Autodesk Inventor part; units mm, degrees
ref_plane "YZ Plane" through (0, 0, 0) normal (1, 0, 0) x (0, 1, 0)
ref_plane "XZ Plane" through (0, 0, 0) normal (0, 1, 0) x (-1, 0, 0)
ref_plane "XY Plane" through (0, 0, 0) normal (0, 0, 1) x (1, 0, 0)
sketch "草图1" plane through (0, 0, 0) normal (0, 1, 0) x (-1, 0, 0)
  line L0 (125, 245) -> (-125, 245)
  line L1 (-125, 245) -> (-125, -245)
  line L2 (-125, -245) -> (125, -245)
  line L3 (125, -245) -> (125, 245)
  line L4 (0, 3) -> (0, -5)
  line L5 (3.5058, 0) -> (-3.4421, 0)
  line L6 (25, 144) -> (-32, 144)
  line L7 (-32, 144) -> (-32, 87)
  line L8 (-32, 87) -> (25, 87)
  line L9 (25, 87) -> (25, 144)
  line L10 (25, 67) -> (-32, 67)
  line L11 (-32, 67) -> (-32, 10)
  line L12 (-32, 10) -> (25, 10)
  line L13 (25, 10) -> (25, 67)
  line L14 (25, -10) -> (-32, -10)
  line L15 (-32, -10) -> (-32, -67)
  line L16 (-32, -67) -> (25, -67)
  line L17 (25, -67) -> (25, -10)
  line L18 (25, -87) -> (-32, -87)
  line L19 (-32, -87) -> (-32, -144)
  line L20 (-32, -144) -> (25, -144)
  line L21 (25, -144) -> (25, -87)
  line L22 (-66, 100) -> (-95, 100)
  line L23 (-95, 100) -> (-95, 54)
  line L24 (-95, 54) -> (-66, 54)
  line L25 (-66, 54) -> (-66, 100)
  line L26 (-66, -54) -> (-95, -54)
  line L27 (-95, -54) -> (-95, -100)
  line L28 (-95, -100) -> (-66, -100)
  line L29 (-66, -100) -> (-66, -54)
  line L30 (100, 15) -> (70, 15)
  line L31 (70, 15) -> (70, -15)
  line L32 (70, -15) -> (100, -15)
  line L33 (100, -15) -> (100, 15)
  circle A0 centre (65, 182) radius 10
  circle A1 centre (65, -182) radius 10
  circle A2 centre (65, 182) radius 15
  circle A3 centre (80, 182) radius 1.5
  circle A4 centre (57.5, 194.9904) radius 1.5
  circle A5 centre (57.5, 169.0096) radius 1.5
  line L34 (125, 245) -> (0, 245)
  line L35 (0, 245) -> (0, 0)
  line L36 (0, 0) -> (125, 0)
  line L37 (125, 0) -> (125, 245)
  line L38 (-125, 245) -> (0, 245)
  line L39 (0, 245) -> (0, 0)
  line L40 (0, 0) -> (-125, 0)
  line L41 (-125, 0) -> (-125, 245)
  line L42 (-125, -245) -> (0, -245)
  line L43 (0, -245) -> (0, 0)
  line L44 (0, 0) -> (-125, 0)
  line L45 (-125, 0) -> (-125, -245)
  line L46 (125, -245) -> (0, -245)
  line L47 (0, -245) -> (0, 0)
  line L48 (0, 0) -> (125, 0)
  line L49 (125, 0) -> (125, -245)
  circle A6 centre (65, -182) radius 15
  circle A7 centre (80, -182) radius 1.5
  circle A8 centre (57.5, -169.0096) radius 1.5
  circle A9 centre (57.5, -194.9904) radius 1.5
  point P0 (0, -144)
  point P1 (100, 0)
  point P2 (70, 0)
  point P3 (0, -10)
  point P4 (0, -67)
  point P5 (0, -87)
  dimension "d33" = 30
  dimension "d36" = 30
  dimension "d2" = 490
  dimension "d3" = 250
  dimension "d4" = 57
  dimension "d5" = 57
  dimension "d6" = 57
  dimension "d7" = 57
  dimension "d8" = 57
  dimension "d9" = 57
  dimension "d10" = 57
  dimension "d11" = 57
  dimension "d12" = 101
  dimension "d13" = 20
  dimension "d14" = 20
  dimension "d15" = 20
  dimension "d16" = 93
  dimension "d17" = 29
  dimension "d18" = 46
  dimension "d19" = 46
  dimension "d20" = 145
  dimension "d21" = 108
  dimension "d22" = 30
  dimension "d23" = 30
  dimension "d24" = 30
  dimension "d25" = 25
  dimension "d26" = 230
  dimension "d27" = 20
  dimension "d28" = 63
  dimension "d29" = 60
  dimension "d30" = 20
  dimension "d31" = 63
  dimension "d32" = 60
  dimension "d34" = 3
  dimension "d35" = 360
  dimension "d37" = 3
  dimension "d40" = 360
extrude "拉伸1" add sketch "草图1" along normal blind 10 contours L3 L2 L43 L20 L21 L18 L16 L17 L14 L4 L5 L36 L31 L32 L33 | A7 A6 A9 A8
sketch "草图2" plane through (0, 0, 0) normal (0, -1, 0) x (1, 0, 0)
  line L0 (-70, 0) -> (0, 0)
  line L1 (-115, -30) -> (-55, -30)
  line L2 (-55, -30) -> (-55, 0)
  line L3 (-55, 0) -> (-115, 0)
  line L4 (-115, 0) -> (-115, -30)
  line L5 (-100, -15) -> (-70, -15)
  line L6 (-100, 0) -> (-100, -15)
  line L7 (-70, -15) -> (-70, 0)
  line L8 (-40, -159) -> (0, -159)
  line L9 (0, -159) -> (0, 0)
  line L10 (0, 0) -> (-40, 0)
  line L11 (-40, 0) -> (-40, -159)
  line L12 (-25, -10) -> (-25, -67)
  line L13 (-25, -144) -> (0, -144)
  circle A0 centre (-65, -182) radius 10
  circle A1 centre (-65, -182) radius 20
  dimension "d44" = 15
  dimension "d45" = 15
  dimension "d46" = 15
  dimension "d47" = 15
  dimension "d48" = 15
  dimension "d49" = 40
extrude "拉伸2" cut sketch "草图2" against normal blind 5 contours L0 L9 L8 L11 | L0 L2 L1 L4 L3 L6 L5 L7 | A1
sketch "草图5" plane through (0, 10, 0) normal (0, 1, 0) x (1, 0, 0)
  line L0 (0, 159) -> (-40, 159)
  line L1 (0, 159) -> (8, 159)
  line L2 (8, 159) -> (8, 245)
  line L3 (8, 245) -> (0, 245)
  line L4 (0, 245) -> (0, 159)
  circle A0 centre (4, 179) radius 2
  circle A1 centre (4, 225) radius 2
  point P0 (0, 0)
  dimension "d64" = 8
  dimension "d65" = 4
  dimension "d67" = 4
  dimension "d68" = 4
  dimension "d70" = 4
  dimension "d73" = 20
  dimension "d76" = 20
extrude "拉伸4" add sketch "草图5" against normal blind 5
properties part number "top_2"
Here's how the part is built. I have some questions about the finished solid (model axes, mm). A direction names the side the tool comes from. Coordinates: 2 decimals unless noted, no trailing zeros. Write each loop counter-clockwise with the first axis right and the second up, starting at its lowest first coordinate (ties: lowest second). Pieces come first, ordered by that corner, then holes.
Item 1: I want a section at A-A on x = -6. Write out the boundary of the cut face in (y, z), and give its area (4 significant figures).
Item 2: Will these pins go through, and if not, where does the flat tip stop? pin 1 (2.5 mm diameter, centred on x = -57.5, z = -169.01, fed in from +Y); pin 2 (5.5 mm diameter, centred on y = 8, z = -4, fed in from +X); pin 3 (1.5 mm diameter, centred on y = 2, z = -22, fed in from +X); pin 4 (5 mm diameter, centred on x = 4, z = -179, fed in from -Y).
Item 3: If I drill on line 1 (X direction, y = 7.95, z = -182); line 2 (Z direction, x = 4, y = 6.65); line 3 (Z direction, x = -80, y = 8.6), over which ranges is the centre line in solid material (lowest first)?
Item 4: I want a section at C-C on y = 8. Write out the boundary of the cut face in (x, z), and give its area (3 significant figures).
Item 5: On a 3-axis mill with a long thin cutter (end or side, diameter ignored), from which of +Z, -Z, +X, -X, +Y, -Y can I reach the whole of each face in a straight line? I mean faces 5 (the flat face through (0, 7, -152)), 6 (the flat face through (-70, 7, -7)), 7 (the flat face through (-115, 2, -15)), 8 (the cylindrical face through (-67.6, 2.46, -162.17)). Say none if no direction works.
Item 6: If we mould it in two halves opening along Z, with no side actions, what happens to faces 1 (the flat face through (-25, 5, -78)), 2 (the flat face through (-20, 2, -159)), 3 (the flat face through (-25, 7, -116)), 4 (the flat face through (-13, 7, -87))? For each: +Z half, -Z half, draft (parallel to the pull), parting line (faces both ways), or undercut.
Item 7: I want a section at D-D on z = -117. Write out the boundary of the cut face in (x, y).
Item 8: I want a section at B-B on x = -65. Write out the boundary of the cut face in (y, z), and give its area (3 significant figures).
Findings below:
1. outline: (0, -245) - (10, -245) - (10, -144) - (5, -144) - (5, -159) - (0, -159) - close; (5, -87) - (10, -87) - (10, -67) - (5, -67) - close; (5, -10) - (10, -10) - (10, 0) - (5, 0) - close
1. area: 1,085 mm2
2. pin 1: passes through
2. pin 2: stops at x = 0
2. pin 3: stops at x = -40
2. pin 4: stops at y = 5
3. line 1: x = -125 to -81.5, -78.5 to -75, -55 to 8
3. line 2: z = -245 to -227, -223 to -181, -177 to -159
3. line 3: z = -245 to -183.5, -180.5 to -15
4. outline: (-125, -245) - (8, -245) - (8, -159) - (0, -159) - (0, -144) - (-25, -144) - (-25, -87) - (0, -87) - (0, -67) - (-25, -67) - (-25, -10) - (0, -10) - (0, 0) - (-70, 0) - (-70, -15) - (-100, -15) - (-100, 0) - (-125, 0) - close; hole circle Ø3 at (-80, -182); hole circle Ø20 at (-65, -182); hole circle Ø3 at (-57.5, -194.99); hole circle Ø3 at (-57.5, -169.01); hole circle Ø4 at (4, -225); hole circle Ø4 at (4, -179)
4. area: 27,700 mm2
5. face 5: +Z, +X, +Y, -Y
5. face 6: +Z, +Y, -Y
5. face 7: +Z, -Y
5. face 8: -Y
6. face 1: draft
6. face 2: +Z half
6. face 3: undercut
6. face 4: undercut
7. outline: (-125, 0) - (-40, 0) - (-40, 5) - (-25, 5) - (-25, 10) - (-125, 10) - close
8. outline: (0, -245) - (10, -245) - (10, -192) - (5, -192) - (5, -202) - (0, -202) - close; (0, -162) - (5, -162) - (5, -172) - (10, -172) - (10, 0) - (5, 0) - (5, -30) - (0, -30) - close
8. area: 2,000 mm2
